Could you check a few things on this model? Use its own coordinates, in mm. Coordinates: 2 decimals unless noted, no trailing zeros. Write each loop counter-clockwise with the first axis right and the second up, starting at its lowest first coordinate (ties: lowest second). Pieces come first, ordered by that corner, then holes. Notation, with made-up numbers: M 38,84 L 71,84 A21 cw 71,122 Z; hole C -19,-26.75 d11. An arc over 180 degrees is marked long. Write item = value, one per line.
```python
from build123d import *

# Parameters (mm, degrees)
SKETCH1_R           = 2.413
BOSS_EXTRUDE1_DEPTH = 3.175
FILLET1_R           = 3.175


with BuildPart() as part:
    # Sketch1 → Boss-Extrude1 (new body)
    with BuildSketch(Plane.XY):
        Polygon((0, 0), (101.6, 0), (101.6, 50.8), (50.8, 50.8), (50.8, 101.6), (0, 101.6), align=None)
        with Locations((12.7, 88.9)):
            Circle(SKETCH1_R, mode=Mode.SUBTRACT)
        with Locations((38.1, 88.9)):
            Circle(SKETCH1_R, mode=Mode.SUBTRACT)
        with Locations((38.1, 63.5)):
            Circle(SKETCH1_R, mode=Mode.SUBTRACT)
        with Locations((12.7, 63.5)):
            Circle(SKETCH1_R, mode=Mode.SUBTRACT)
        with Locations(Location((38.1, 12.7, 0), (0, 0, 180))):
            Circle(SKETCH1_R, mode=Mode.SUBTRACT)
        with Locations(Location((38.1, 38.1, 0), (0, 0, 180))):
            Circle(SKETCH1_R, mode=Mode.SUBTRACT)
        with Locations(Location((12.7, 38.1, 0), (0, 0, 180))):
            Circle(SKETCH1_R, mode=Mode.SUBTRACT)
        with Locations(Location((12.7, 12.7, 0), (0, 0, 180))):
            Circle(SKETCH1_R, mode=Mode.SUBTRACT)
        with Locations((88.9, 12.7)):
            Circle(SKETCH1_R, mode=Mode.SUBTRACT)
        with Locations((63.5, 12.7)):
            Circle(SKETCH1_R, mode=Mode.SUBTRACT)
        with Locations((63.5, 38.1)):
            Circle(SKETCH1_R, mode=Mode.SUBTRACT)
        with Locations((88.9, 38.1)):
            Circle(SKETCH1_R, mode=Mode.SUBTRACT)
    extrude(amount=BOSS_EXTRUDE1_DEPTH)

    # Fillet1
    fillet1_edges = [part.edges().sort_by_distance(p)[0] for p in [
        (0, 101.6, 1.5875),
        (50.8, 101.6, 1.5875),
        (50.8, 50.8, 1.5875),
        (101.6, 50.8, 1.5875),
        (101.6, 0, 1.5875),
        (0, 0, 1.5875),
    ]]
    fillet(fillet1_edges, radius=FILLET1_R)


solid = part.part
```
Item 1: I'm going to push flat-ended pins straight in: P1, Ø1.6, axis at y = 83, z = 1.5, coming from the +X side; P2, Ø1, axis at x = 80, z = 2, coming from the +Y side. Where does each tip first touch, or does it pass through?
Numbers:
P1 = 50.8
P2 = 50.8
Item 2: If we mould it in two halves opening along Y, with no side actions, what happens to faces 1 (the face through (91.202, 38.825, 1.565)), 2 (the face through (101.6, 25, 2)), 3 (the face through (77, 50.8, 2)), 4 (the face through (0.95, 0.91, 1.61))? For each: pulls with the +Y half, pulls with the -Y half, needs draft (parallel to the pull), parting line crosses it, or undercut.
Numbers:
face_1 = undercut
face_2 = needs draft
face_3 = pulls with the +Y half
face_4 = pulls with the -Y half
Item 3: Imagine slicing it at C-C (z = 1.7). State how many separate pieces and enclosed holes the cut face has, and give its area (3 significant figures).
Numbers:
separate_pieces = 1
enclosed_holes = 12
area = 7,510 mm²
Item 4: Imagine slicing it at B-B (y = 88.9). Write out the boundary of the cut face in (x, z) (3 decimals), and give its area (3 significant figures).
Numbers:
outline = M 0,0 L 10.287,0 L 10.287,3.175 L 0,3.175 Z; M 15.113,0 L 35.687,0 L 35.687,3.175 L 15.113,3.175 Z; M 40.513,0 L 50.8,0 L 50.8,3.175 L 40.513,3.175 Z
area = 131 mm²
Item 5: Imagine slicing it at A-A (x = 12.7). Write out the boundary of the cut face in (y, z) (3 decimals).
Numbers:
outline = M 0,0 L 10.287,0 L 10.287,3.175 L 0,3.175 Z; M 15.113,0 L 35.687,0 L 35.687,3.175 L 15.113,3.175 Z; M 40.513,0 L 61.087,0 L 61.087,3.175 L 40.513,3.175 Z; M 65.913,0 L 86.487,0 L 86.487,3.175 L 65.913,3.175 Z; M 91.313,0 L 101.6,0 L 101.6,3.175 L 91.313,3.175 Z
Item 6: If I drill on line 1 along Y through (x, z) = (63.5, 1.9); line 2 along Y through (x, z) = (12.7, 0.7); line 3 along Y through (x, z) = (36, 0.35), over which ranges is the centre line in solid material (lowest first)?
Numbers:
line_1 = 0 to 10.29, 15.11 to 35.69, 40.51 to 50.8
line_2 = 0 to 10.29, 15.11 to 35.69, 40.51 to 61.09, 65.91 to 86.49, 91.31 to 101.6
line_3 = 0 to 11.51, 13.89 to 36.91, 39.29 to 62.31, 64.69 to 87.71, 90.09 to 101.6
